The drawing under review shows one solid part. Ordinate dimensions are in mm from its lowest x, y, z. A direction names the side the tool comes from. Give positions to 0.01 mm unless a question says otherwise; leave off trailing zeros. Loops run counter-clockwise (first coordinate to the right, second up) from the corner with the lowest first, then second, coordinate; pieces in that order, holes last.
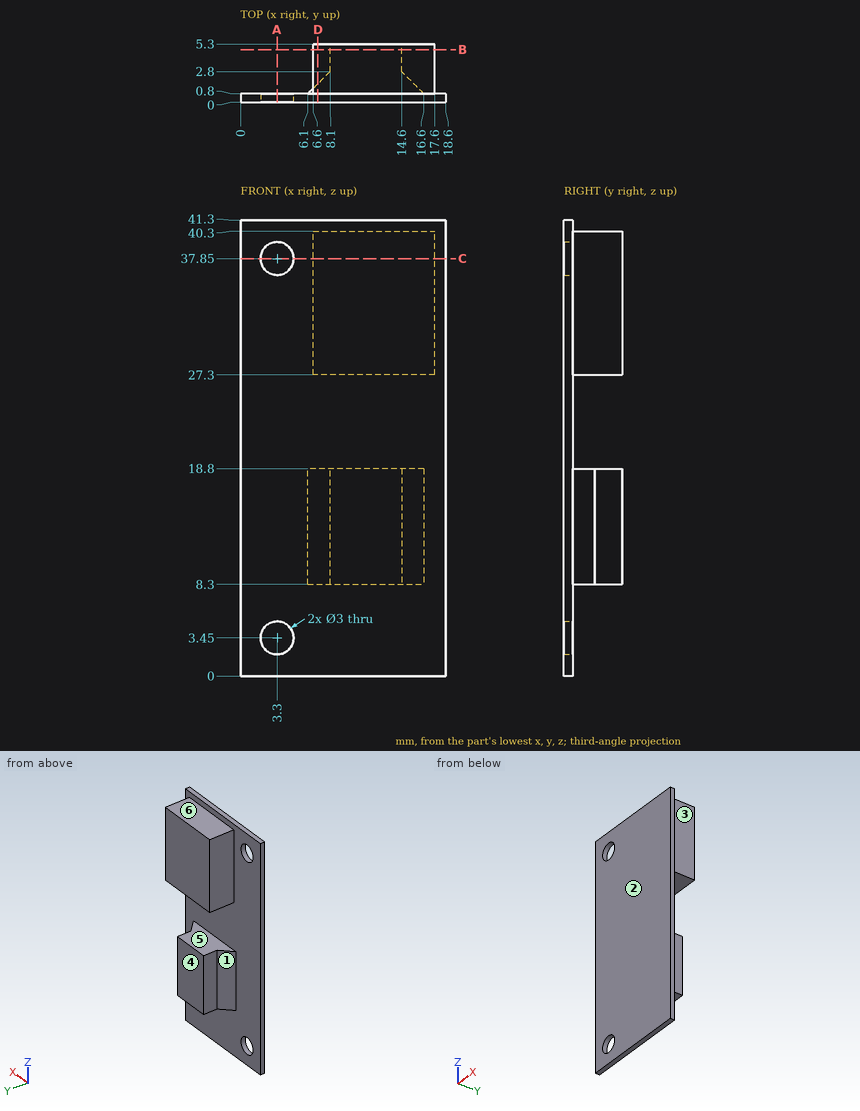
Item 1: Take a section at D-D on x = 7. Give the boundary of the cut face in (y, z), and give its area (3 significant figures).
Answer:
outline: (0, 0) - (0.8, 0) - (0.8, 8.3) - (1.7, 8.3) - (1.7, 18.8) - (0.8, 18.8) - (0.8, 27.3) - (5.3, 27.3) - (5.3, 40.3) - (0.8, 40.3) - (0.8, 41.3) - (0, 41.3) - close
area: 101 mm2
Item 2: Tool access review of the marked faces 1, 2 and 3: name each direction out of +Z, -Z, +X, -X, +Y, -Y from which nothing blocks a thin tool from reaching the whole face with its end or side.
Answer:
face 1: -Z, -X, +Y
face 2: +Z, -Z, +X, -X, -Y
face 3: +Z, -Z, +X, +Y
Item 3: Take a section at C-C on z = 37.85. Give the boundary of the cut face in (x, y), and give its area (3 significant figures).
Answer:
outline: (0, 0) - (1.8, 0) - (1.8, 0.8) - (0, 0.8) - close; (4.8, 0) - (18.6, 0) - (18.6, 0.8) - (17.6, 0.8) - (17.6, 5.3) - (6.6, 5.3) - (6.6, 0.8) - (4.8, 0.8) - close
area: 62.0 mm2
Item 4: For L1, parallel to Z at x = 3.3, y = 0.3; L2, parallel to X at y = 0.2, z = 3.45; L3, parallel to Z at x = 8.5, y = 1.7, list the stretches that pass through material, from the lowest coordinate up.
Answer:
L1: z = 0 to 1.95, 4.95 to 36.35, 39.35 to 41.3
L2: x = 0 to 1.8, 4.8 to 18.6
L3: z = 8.3 to 18.8, 27.3 to 40.3
Item 5: Clearance check with flat-ended pins moving along their axes: pin 1 Ø2.5 at (x, y) = (9, 2) entering from +Z; pin 2 Ø3 at (x, y) = (9, 4.5) entering from +Z; pin 3 Ø1.3 at (y, z) = (3.5, 34.5) entering from -X; pin 4 Ø2.5 at (x, y) = (10.5, 3) entering from -Z. State where each tip first meets the part, or that it passes through.
Answer:
pin 1: stops at z = 41.3
pin 2: stops at z = 40.3
pin 3: stops at x = 6.6
pin 4: stops at z = 8.3
Item 6: The part is to be moulded in two halves that separate along Z. For the marked faces 4, 5 and 6, say which applies: released by +Z, released by -Z, zero draft, split by the parting line, or undercut.
Answer:
face 4: zero draft
face 5: undercut
face 6: released by +Z
Item 7: Take a section at A-A on x = 3.3. Give the boundary of the cut face in (y, z), and give its area (3 significant figures).
Answer:
outline: (0, 0) - (0.8, 0) - (0.8, 1.95) - (0, 1.95) - close; (0, 4.95) - (0.8, 4.95) - (0.8, 36.35) - (0, 36.35) - close; (0, 39.35) - (0.8, 39.35) - (0.8, 41.3) - (0, 41.3) - close
area: 28.2 mm2
Item 8: Take a section at B-B on y = 4.8. Give the boundary of the cut face in (x, z).
Answer:
outline: (6.6, 27.3) - (17.6, 27.3) - (17.6, 40.3) - (6.6, 40.3) - close; (8.1, 8.3) - (14.6, 8.3) - (14.6, 18.8) - (8.1, 18.8) - close
